Part model, mm, in its own coordinate system. Round coordinates to 2 decimals unless told otherwise and drop trailing zeros. Write each loop counter-clockwise with the first axis right and the second up, starting at its lowest first coordinate (ties: lowest second). Pieces come first, ordered by that corner, then holes. Notation, with made-up numbers: M 78.25,41 L 86.25,41 A36 cw 86.25,80 Z; hole C 11.5,19 d3. An arc over 180 degrees is marked long. Use a Markdown table: item, result. Add a question column.
1) Slice it at D-D on x = 12. Write the cut outline in (y, z), plus the area to 3 significant figures.
2) Slice it at B-B on y = 8. Write the cut outline in (x, z).
3) Drop flat-ended pins along their axis: P1, Ø10, axis at x = -25.5, y = 12.5, coming from the -Z side; P2, Ø1, axis at x = 17, z = -0.5, coming from the +Y side; P3, Ø1, axis at x = -51, z = -0.5, coming from the -Y side; P4, Ø1, axis at x = -21.5, z = 0.5, coming from the +Y side. Give the stop position or say it passes through.
4) Slice it at C-C on x = -20. Write the cut outline in (y, z).
5) Wall check: probe 1 along X at (y, z) = (6, 0.5); probe 2 along Y at (x, z) = (-55.5, -0.6); probe 3 along Y at (x, z) = (-47, -0.4). Give the ranges that are in metal, low to high.
6) Slice it at A-A on z = -0.55. Write the cut outline in (x, y).
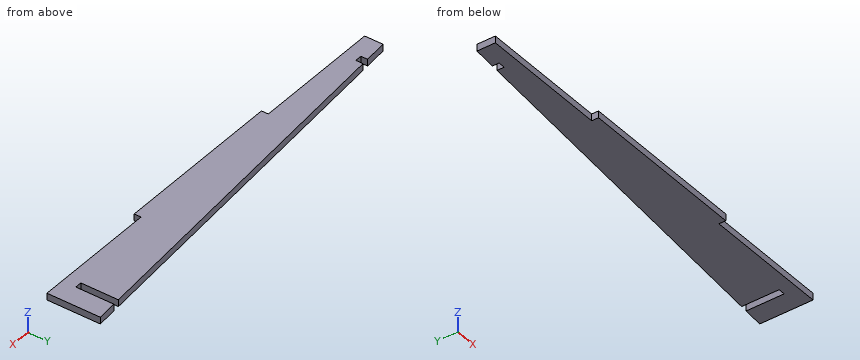
Autodesk Inventor part; units mm, degrees
ref_plane "YZ Plane" through (0, 0, 0) normal (1, 0, 0) x (0, 1, 0)
ref_plane "XZ Plane" through (0, 0, 0) normal (0, 1, 0) x (-1, 0, 0)
ref_plane "XY Plane" through (0, 0, 0) normal (0, 0, 1) x (1, 0, 0)
sketch "Sketch1" plane through (0, 0, 0) normal (0, 0, 1) x (1, 0, 0)
  line L0 (-64, 50) -> (64, 50)
  line L1 (64, 50) -> (64, 0)
  line L2 (64, 0) -> (-64, 0)
  line L3 (-64, 0) -> (-64, 50)
  line L4 (-25, 0) -> (25, 0)
  line L5 (25, 0) -> (25, -2)
  line L6 (25, -2) -> (-25, -2)
  line L7 (-25, -2) -> (-25, 0)
  point P0 (0, 0)
  point P1 (0, 0)
  dimension "d0" = 50
  dimension "d1" = 128
  dimension "d2" = 2
  dimension "d3" = 50
extrude "Extrusion1" add sketch "Sketch1" along normal mid plane 2
sketch "Sketch2" plane through (0, 0, 1) normal (0, 0, 1) x (1, 0, 0)
  line L0 (53.9533, 19.1647) -> (54.2948, 15.001)
  line L1 (54.2948, 15.001) -> (-55.3369, 6.0072)
  line L2 (-55.3369, 6.0072) -> (-55.6784, 10.1709)
  line L3 (-55.6784, 10.1709) -> (53.9533, 19.1647)
  line L4 (62.1376, 13.5765) -> (61.7855, 17.8679)
  line L5 (-63.1946, 7.615) -> (-62.8426, 3.3235)
  point P0 (0, 0)
sketch "Sketch3" plane through (0, 0, 1) normal (0, 0, 1) x (1, 0, 0)
  line L0 (-63.1946, 7.615) -> (-62.8426, 3.3235) construction
  line L1 (62.1376, 13.5765) -> (61.7855, 17.8679) construction
  line L2 (54.2948, 15.001) -> (-55.3369, 6.0072) construction
  line L3 (-62.8426, 5.3914) -> (61.9691, 15.6306)
  line L4 (-62.8426, 5.3914) -> (-62.8426, 0)
  line L5 (-62.8426, 0) -> (-72.8426, 0)
  line L6 (-72.8426, 0) -> (-72.8426, 60)
  line L7 (-72.8426, 60) -> (71.9691, 60)
  line L8 (71.9691, 60) -> (71.9691, 0)
  line L9 (71.9691, 0) -> (61.9691, 0)
  line L10 (61.9691, 0) -> (61.9691, 15.6306)
  point P0 (0, 0)
  dimension "d6" = 10
  dimension "d7" = 60
  dimension "d8" = 10
extrude "Extrusion2" cut sketch "Sketch3" against normal through all
sketch "Sketch4" plane through (0, 0, 1) normal (0, 0, 1) x (1, 0, 0)
  line L0 (56, 14.7768) -> (56, 0)
  line L1 (54, 14.7768) -> (56, 14.7768)
  line L2 (54, 0) -> (54, 14.7768)
  line L3 (56, 0) -> (54, 0)
  line L4 (-54, 5.783) -> (-54, 0)
  line L5 (-56, 5.783) -> (-54, 5.783)
  line L6 (-56, 0) -> (-56, 5.783)
  line L7 (-54, 0) -> (-56, 0)
  point P0 (0, 0)
sketch "Sketch5" plane through (0, 0, 1) normal (0, 0, 1) x (1, 0, 0)
  line L0 (-56, 0) -> (-56, 5.783) construction
  line L1 (-54, 5.783) -> (-54, 0) construction
  line L2 (54, 0) -> (54, 14.7768) construction
  line L3 (56, 14.7768) -> (56, 0) construction
  line L4 (-54, 4) -> (-56, 4)
  line L5 (-56, 4) -> (-56, 24)
  line L6 (-56, 24) -> (-54, 24)
  line L7 (-54, 24) -> (-54, 4)
  line L8 (56, 24) -> (54, 24)
  line L9 (54, 24) -> (54, 4)
  line L10 (54, 4) -> (56, 4)
  line L11 (56, 4) -> (56, 24)
  line L12 (-62.8426, 0) -> (-25, 0)
  line L13 (25, 0) -> (61.9691, 0)
  point P0 (0, 0)
  dimension "d11" = 4
  dimension "d12" = 20
  dimension "d13" = 4
  dimension "d14" = 20
extrude "Extrusion3" cut sketch "Sketch5" against normal through all
properties part number "angle_plate_long_short"
Entries:
| question | item | result |
|---|---|---|
| 1 | outline | M -2,-1 L 11.53,-1 L 11.53,1 L -2,1 Z |
| 1 | area | 27.1 mm^2 |
| 2 | outline | M -31.04,-1 L 54,-1 L 54,1 L -31.04,1 Z; M 56,-1 L 61.97,-1 L 61.97,1 L 56,1 Z |
| 3 | P1 | stops at z = -1 |
| 3 | P2 | stops at y = 11.98 |
| 3 | P3 | stops at y = 0 |
| 3 | P4 | stops at y = 8.82 |
| 4 | outline | M -2,-1 L 8.91,-1 L 8.91,1 L -2,1 Z |
| 5 | probe 1 | x = -54 to 54, 56 to 61.97 |
| 5 | probe 2 | y = 0 to 4 |
| 5 | probe 3 | y = 0 to 6.69 |
| 6 | outline | M -62.84,0 L -25,0 L -25,-2 L 25,-2 L 25,0 L 61.97,0 L 61.97,15.63 L 56,15.14 L 56,4 L 54,4 L 54,14.98 L -54,6.12 L -54,4 L -56,4 L -56,5.95 L -62.84,5.39 Z |
